Here's the drawing with two shaded views (mm, measured from the low corner). I have some questions. A direction names the side the tool comes from. Coordinates: 2 decimals unless noted, no trailing zeros. Write each loop counter-clockwise with the first axis right and the second up, starting at its lowest first coordinate (ties: lowest second). Pieces come first, ordered by that corner, then holes. Notation, with made-up numbers: M 2,-34 L 11,-34 A14 ccw 11,-11 Z; hole C 18.5,13.5 d2. An arc over 180 degrees is marked long. Use one line per item in the form item = value. Start each with the question number.
1. I want a section at D-D, the plane y = 29. List the corners of the cut face in (x, z) for me.
2. I want a section at B-B, the plane y = 39. List the corners of the cut face in (x, z) for me.
3. I want a section at A-A, the plane x = 36.5. List the corners of the cut face in (y, z) for me, plus the area to 3 significant figures.
4. Thinking about a two-plate mould opening in Y: for the marked faces 1, 2 and 3, which applies, released by +Y, released by -Y, zero draft, split by the parting line, or undercut?
5. I want a section at C-C, the plane z = 2.2. Count the separate pieces of the cut face and the enclosed holes in it, plus the area to 3 significant figures.
6. Please list where these lines run through material, in increasing order: line 1 along Y through (x, z) = (35, 2.3); line 2 along Y through (x, z) = (30.5, 1.25); line 3 along X through (y, z) = (21, 5.45). Write a range as [from, to].
7. I'm going to push flat-ended pins straight in: pin 1 Ø1.5 at (y, z) = (21, 4) entering from -X; pin 2 Ø3 at (y, z) = (29.5, 4) entering from -X; pin 3 Ø1.8 at (y, z) = (28, 4) entering from +X; pin 4 Ø1.8 at (x, z) = (65.5, 3.5) entering from -Y. Where does each tip first touch, or does it pass through?
8. On a 3-axis mill with a long thin cutter (end or side, diameter ignored), from which of +Z, -Z, +X, -X, +Y, -Y can I reach the whole of each face in a straight line? I mean the marked faces 4, 5 and 6. Say none if no direction works.
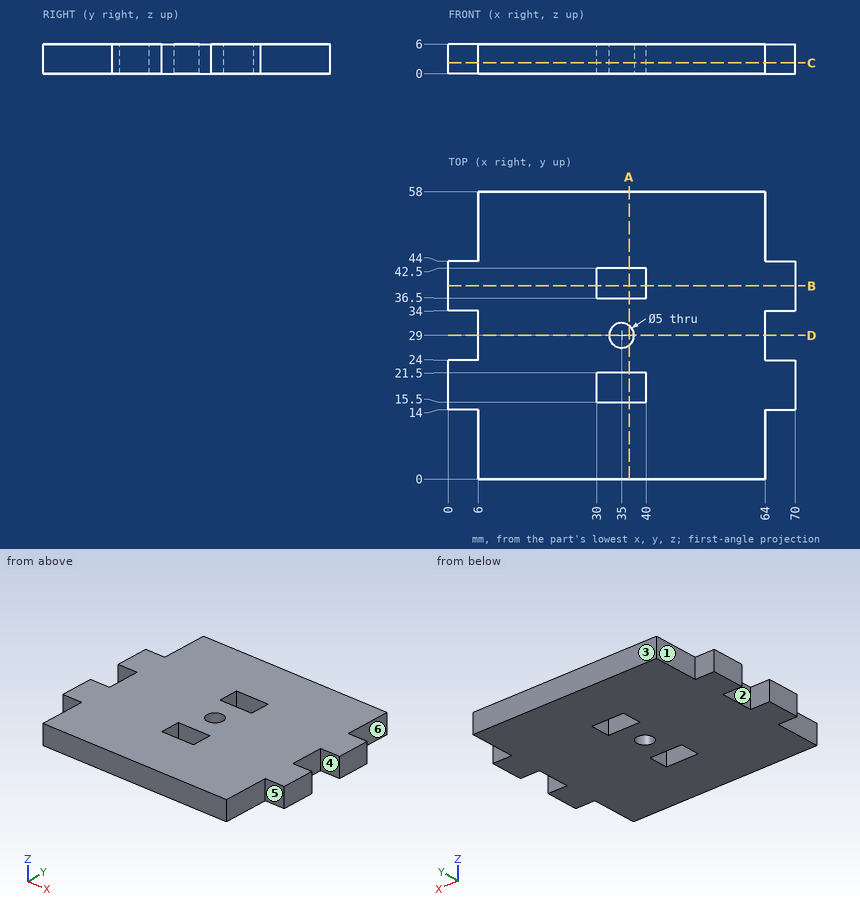
Answer list:
q1.outline = M 6,0 L 32.5,0 L 32.5,6 L 6,6 Z; M 37.5,0 L 64,0 L 64,6 L 37.5,6 Z
q2.outline = M 0,0 L 30,0 L 30,6 L 0,6 Z; M 40,0 L 70,0 L 70,6 L 40,6 Z
q3.outline = M 0,0 L 15.5,0 L 15.5,6 L 0,6 Z; M 21.5,0 L 27,0 L 27,6 L 21.5,6 Z; M 31,0 L 36.5,0 L 36.5,6 L 31,6 Z; M 42.5,0 L 58,0 L 58,6 L 42.5,6 Z
q3.area = 252 mm²
q4.face_1 = zero draft
q4.face_2 = undercut
q4.face_3 = released by +Y
q5.separate_pieces = 1
q5.enclosed_holes = 3
q5.area = 3,460 mm²
q6.line_1 = [0, 15.5], [21.5, 26.5], [31.5, 36.5], [42.5, 58]
q6.line_2 = [0, 15.5], [21.5, 36.5], [42.5, 58]
q6.line_3 = [0, 30], [40, 70]
q7.pin_1 = 0
q7.pin_2 = 6
q7.pin_3 = 64
q7.pin_4 = 14
q8.face_4 = +Z, -Z, +X
q8.face_5 = +Z, -Z, +X, -Y
q8.face_6 = +Z, -Z, +X, +Y
